Autodesk Inventor part; units mm, degrees
ref_plane "YZ Plane" through (0, 0, 0) normal (1, 0, 0) x (0, 1, 0)
ref_plane "XZ Plane" through (0, 0, 0) normal (0, 1, 0) x (-1, 0, 0)
ref_plane "XY Plane" through (0, 0, 0) normal (0, 0, 1) x (1, 0, 0)
sketch "Sketch1" plane through (0, 0, 0) normal (0, 1, 0) x (-1, 0, 0)
  line L0 (-44.45, 77.47) -> (44.45, 77.47)
  line L1 (44.45, 77.47) -> (44.45, -77.47)
  line L2 (44.45, -77.47) -> (-44.45, -77.47)
  line L3 (-44.45, -77.47) -> (-44.45, 77.47)
  line L4 (-44.45, 77.47) -> (44.45, -77.47) construction
  line L5 (44.45, 77.47) -> (-44.45, -77.47) construction
  point P0 (0, 0)
  dimension "d0" = 154.94
  dimension "d1" = 88.9
extrude "Extrusion1" add sketch "Sketch1" along normal blind 4.7625
fillet "Fillet1" radius 3.175 4 edges at (44.45, 2.3813, 77.47) (-44.45, 2.3813, 77.47) (44.45, 2.3813, -77.47) (-44.45, 2.3813, -77.47)
sketch "Sketch9" plane through (41.275, 0, -77.47) normal (0, 0, -1) x (-1, 0, 0)
  line L0 (0, 4.7625) -> (82.55, 4.7625)
  line L1 (41.275, 0) -> (47.625, 0)
  line L2 (47.625, 0) -> (47.625, 4.7625)
  line L3 (47.625, 4.7625) -> (41.275, 4.7625)
  line L4 (41.275, 4.7625) -> (41.275, 0)
  dimension "d40" = 6.35
sketch "Sketch10" plane through (-44.45, 0, -74.295) normal (-1, 0, 0) x (0, 0, 1)
  line L0 (0, 4.7625) -> (148.59, 4.7625)
  line L1 (74.295, 0) -> (80.645, 0)
  line L2 (80.645, 0) -> (80.645, 4.7625)
  line L3 (80.645, 4.7625) -> (74.295, 4.7625)
  line L4 (74.295, 4.7625) -> (74.295, 0)
  dimension "d41" = 6.35
sketch "Sketch11" plane through (44.45, 0, 74.295) normal (1, 0, 0) x (0, 0, -1)
  line L0 (148.59, 4.7625) -> (0, 4.7625)
  line L1 (74.295, 0) -> (80.645, 0)
  line L2 (80.645, 0) -> (80.645, 4.7625)
  line L3 (80.645, 4.7625) -> (74.295, 4.7625)
  line L4 (74.295, 4.7625) -> (74.295, 0)
  dimension "d42" = 6.35
sketch "Sketch12" plane through (-41.275, 0, 77.47) normal (0, 0, 1) x (1, 0, 0)
  line L0 (82.55, 4.7625) -> (0, 4.7625)
  line L1 (41.275, 0) -> (47.625, 0)
  line L2 (47.625, 0) -> (47.625, 4.7625)
  line L3 (47.625, 4.7625) -> (41.275, 4.7625)
  line L4 (41.275, 4.7625) -> (41.275, 0)
  dimension "d43" = 6.35
extrude "Extrusion8" add sketch "Sketch11" along normal blind 25.4
extrude "Extrusion9" add sketch "Sketch12" along normal blind 25.4
extrude "Extrusion10" add sketch "Sketch10" along normal blind 25.4
extrude "Extrusion11" add sketch "Sketch9" along normal blind 25.4
properties part number "iceTubeClockTop"
Read the model definition and answer for the solid it produces. Units are mm, in the model's axes. A direction names the side the tool comes from. Give positions to 0.01 mm unless a question says otherwise; leave off trailing zeros. Loops run counter-clockwise (first coordinate to the right, second up) from the corner with the lowest first, then second, coordinate; pieces in that order, holes last. Notation, with made-up numbers: M 85.5,1.5 L 116.5,1.5 A20 cw 116.5,19.5 Z; hole C 77,6.25 d11. An arc over 180 degrees is marked long. Write each question's results on one line, items separated by ' | '.
1. Section A-A on y = 0.9 is taken. Give the vertices of the cut face in (x, z) (3 decimals), plus the area to 3 significant figures.
Values:
outline: M -69.85,0 L -44.45,0 L -44.45,-74.295 A3.175 ccw -41.275,-77.47 L -6.35,-77.47 L -6.35,-102.87 L 0,-102.87 L 0,-77.47 L 41.275,-77.47 A3.175 ccw 44.45,-74.295 L 44.45,-6.35 L 69.85,-6.35 L 69.85,0 L 44.45,0 L 44.45,74.295 A3.175 ccw 41.275,77.47 L 6.35,77.47 L 6.35,102.87 L 0,102.87 L 0,77.47 L -41.275,77.47 A3.175 ccw -44.45,74.295 L -44.45,6.35 L -69.85,6.35 Z | area: 14,400 mm^2
2. Straight lines are drawn through the part: line 1 (X direction, y = 0.25, z = 93); line 2 (Z direction, x = -16, y = 2.3); line 3 (Z direction, x = -2.5, y = 0.95). For each, find the intervals that lie inside material, in ascending order. Write a range as [from, to].
Values:
line 1: x = [0, 6.35] | line 2: z = [-77.47, 77.47] | line 3: z = [-102.87, 77.47]
3. Given pin 1 (1.5 mm diameter, centred on y = 1, z = -46.5, fed in from +X); pin 2 (2.5 mm diameter, centred on y = 2.5, z = -84.5, fed in from +X); pin 3 (2.5 mm diameter, centred on x = -61.5, y = 3, fed in from +Z), each flat-ended and moving along its own axis, determine where each tip first touches the part or whether it passes through.
Values:
pin 1: stops at x = 44.45 | pin 2: stops at x = 0 | pin 3: stops at z = 6.35
4. A tool of negligible diameter and unlimited length cuts with its end or side. For faces 1 (the face through (-6.35, 2, -90)), 2 (the face through (-44.45, 2, 41)), 3 (the face through (6.35, 2, 90)), from which of +Z, -Z, +X, -X, +Y, -Y can it reach the whole face along a straight path? Write none if from no direction.
Values:
face 1: -Z, -X, +Y, -Y | face 2: +Z, -X, +Y, -Y | face 3: +Z, +X, +Y, -Y
5. Section C-C on z = 69.5 is taken. Give the vertices of the cut face in (x, y).
Values:
outline: M -44.45,0 L 44.45,0 L 44.45,4.76 L -44.45,4.76 Z
6. Section B-B on x = -9.5 is taken. Give the vertices of the cut face in (y, z), plus the area to 3 significant figures.
Values:
outline: M 0,-77.47 L 4.76,-77.47 L 4.76,77.47 L 0,77.47 Z | area: 738 mm^2
